The model under review builds one solid part; all positions refer to its coordinate system, in mm. Face numbers are marked on the shaded views. A direction names the side the tool comes from. Coordinates: 2 decimals unless noted, no trailing zeros. Loops run counter-clockwise (first coordinate to the right, second up) from the corner with the lowest first, then second, coordinate; pieces in that order, holes last. Notation, with made-up numbers: M 37.5,87 L 59.5,87 A25 cw 59.5,110 Z; hole C 82.25,17 d3. An arc over 180 degrees is marked long. Use CSV: the item, a comma, the result in double quotes. Start each with the question number.
1. Add section D-D, the plane z = 1.25. Write out the cut boundary in (x, y), then the cut area to 3 significant figures.
2. For L1, parallel to Y at x = 3, z = 3; L2, parallel to Z at x = -0.25, y = 23.75; L3, parallel to Z at x = 4.25, y = 16.25, list the stretches that pass through material, from the lowest coordinate up.
3. Tool access review of the marked faces 5, 6 and 7: name each direction out of +Z, -Z, +X, -X, +Y, -Y from which nothing blocks a thin tool from reaching the whole face with its end or side.
4. Draft analysis for pull direction X (two halves, no side actions). For the marked faces 1, 2, 3 and 4, state which applies: +X half, -X half, draft (parallel to the pull), parting line (faces both ways), or undercut.
5. Add section A-A, the plane z = 0. Write out the cut boundary in (x, y).
6. Add section C-C, the plane y = 20.25. Write out the cut boundary in (x, z).
7. Add section B-B, the plane x = 0. Write out the cut boundary in (y, z), then the cut area to 3 significant figures.
8. Clearance check with flat-ended pins moving along their axes: P1, Ø1, axis at y = 22.5, z = -0.5, coming from the +X side; P2, Ø6, axis at x = 4, y = 15.5, coming from the -Z side; P3, Ø1, axis at y = 21.5, z = 0, coming from the -X side. State where each tip first meets the part, or that it passes through.
from build123d import *

# Parameters (mm, degrees)
SKETCH1_R           = 5
BOSS_EXTRUDE1_DEPTH = 20
SKETCH2_W           = 2
SKETCH2_H           = 2
BOSS_EXTRUDE2_DEPTH = 10
SKETCH3_R           = 5
CUT_EXTRUDE1_DEPTH  = 32


with BuildPart() as part:
    # Sketch1 → Boss-Extrude1 (new body)
    with BuildSketch(Plane(origin=(0, 0, 0), x_dir=(1, 0, 0), z_dir=(0, 1, 0))):
        with Locations(Location((0, 0, 0), (0, 0, 270))):
            Circle(SKETCH1_R)
    extrude(amount=BOSS_EXTRUDE1_DEPTH)

    # Sketch2 → Boss-Extrude2 (add)
    with BuildSketch(Plane(origin=(0, 20, 0), x_dir=(1, 0, 0), z_dir=(0, 1, 0))):
        Rectangle(SKETCH2_W, SKETCH2_H)
    extrude(amount=BOSS_EXTRUDE2_DEPTH)

    # Sketch3 → Cut-Extrude1 (cut, through all)
    with BuildSketch(Plane.XY.offset(1)):
        with Locations((0, 30)):
            Circle(SKETCH3_R)
    extrude(amount=-CUT_EXTRUDE1_DEPTH, mode=Mode.SUBTRACT)


solid = part.part
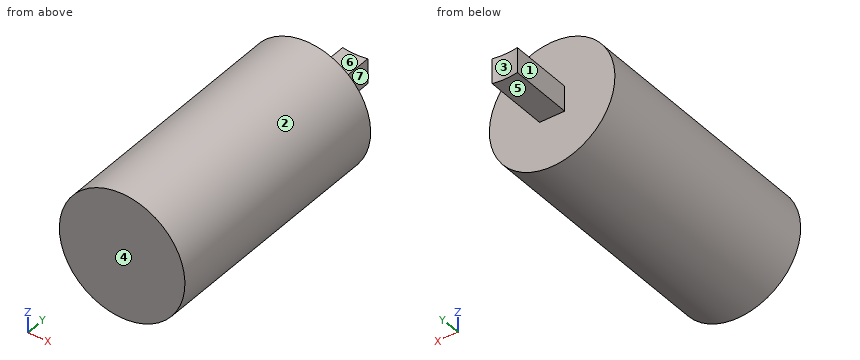
Computed:
1,outline,"M -4.84,0 L 4.84,0 L 4.84,20 L -4.84,20 Z"
1,area,"194 mm^2"
2,L1,"y = 0 to 20"
2,L2,"z = -1 to 1"
2,L3,"z = -2.63 to 2.63"
3,face 5,"-Z, +X, -X, +Y"
3,face 6,"+Z, +X, -X, +Y"
3,face 7,"+Z, -Z, +X, +Y"
4,face 1,"-X half"
4,face 2,"parting line"
4,face 3,"undercut"
4,face 4,"draft"
5,outline,"M -5,0 L 5,0 L 5,20 L 1,20 L 1,25.1 A5 cw -1,25.1 L -1,20 L -5,20 Z"
6,outline,"M -1,-1 L 1,-1 L 1,1 L -1,1 Z"
7,outline,"M 0,-5 L 20,-5 L 20,-1 L 25,-1 L 25,1 L 20,1 L 20,5 L 0,5 Z"
7,area,"210 mm^2"
8,P1,"stops at x = 1"
8,P2,"stops at z = -4.9"
8,P3,"stops at x = -1"
